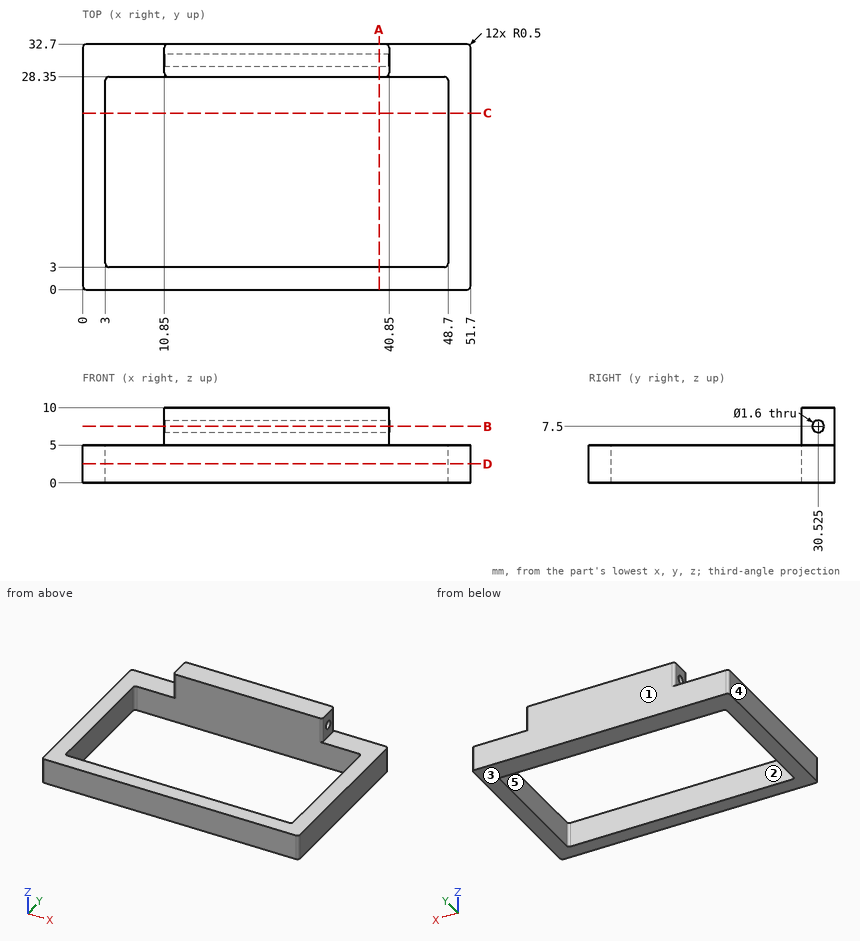
Geometry check sheet. Reference: drawing and pictorial views, mm from the part's lowest x, y, z. A direction names the side the tool comes from. Give positions to 0.01 mm unless a question says otherwise; leave off trailing zeros. Write each loop counter-clockwise with the first axis right and the second up, starting at its lowest first coordinate (ties: lowest second). Pieces come first, ordered by that corner, then holes. Notation, with made-up numbers: (-5, -38) - (28, -38) arc R17 cw to (28, -33) - close; hole circle Ø2 at (76, -36.75). An arc over 180 degrees is marked (long way). Put each result on its own line as item: value.
Q1. Mould release check, pull along Y, two halves, no side actions. Record for the marked faces 1, 2 and 3: released by +Y, released by -Y, zero draft, split by the parting line, or undercut.
Result:
face 1: released by +Y
face 2: undercut
face 3: zero draft
Q2. Section check B-B on z = 7.5. Record the cut outline in (x, y) (3 decimals).
Result:
outline: (10.85, 28.85) arc R0.5 ccw to (11.35, 28.35) - (40.35, 28.35) arc R0.5 ccw to (40.85, 28.85) - (40.85, 29.725) - (10.85, 29.725) - close; (10.85, 31.325) - (40.85, 31.325) - (40.85, 32.2) arc R0.5 ccw to (40.35, 32.7) - (11.35, 32.7) arc R0.5 ccw to (10.85, 32.2) - close
Q3. Section check A-A on x = 39.5. Record the cut outline in (y, z) (3 decimals).
Result:
outline: (0, 0) - (3, 0) - (3, 5) - (0, 5) - close; (28.35, 0) - (32.7, 0) - (32.7, 10) - (28.35, 10) - close; hole circle Ø1.6 at (30.525, 7.5)
Q4. Scan lines: probe 1 along Y at (x, z) = (37, 0.5); probe 2 along X at (y, z) = (8, 3.5); probe 3 along Y at (x, z) = (27.5, 9.5). Record each from-to range of solid material in increasing order. Write a range as from..to.
Result:
probe 1: 0..3, 28.35..32.7
probe 2: 0..3, 48.7..51.7
probe 3: 28.35..32.7
Q5. Section check C-C on y = 23.5. Record the cut outline in (x, z), and give its area (3 significant figures).
Result:
outline: (0, 0) - (3, 0) - (3, 5) - (0, 5) - close; (48.7, 0) - (51.7, 0) - (51.7, 5) - (48.7, 5) - close
area: 30.0 mm2
Q6. Section check D-D on z = 2.5. Record the cut outline in (x, y), and give its area (3 significant figures).
Result:
outline: (0, 0.5) arc R0.5 ccw to (0.5, 0) - (51.2, 0) arc R0.5 ccw to (51.7, 0.5) - (51.7, 32.2) arc R0.5 ccw to (51.2, 32.7) - (0.5, 32.7) arc R0.5 ccw to (0, 32.2) - close; hole (3, 3.5) arc R0.5 ccw to (3.5, 3) - (48.2, 3) arc R0.5 ccw to (48.7, 3.5) - (48.7, 27.85) arc R0.5 ccw to (48.2, 28.35) - (3.5, 28.35) arc R0.5 ccw to (3, 27.85) - close
area: 532 mm2
Q7. Depth check by flat-ended pin: P1, Ø1.5, axis at x = 19.5, z = 8.5, coming from the -Y side; P2, Ø1, axis at y = 30, z = 8.5, coming from the -X side; P3, Ø4, axis at x = 23.5, y = 5.5, coming from the +Z side; P4, Ø1, axis at y = 30.5, z = 6.5, coming from the +X side. Enter the tip coordinate at first touch or a pass-through.
Result:
P1: y = 28.35
P2: x = 10.85
P3: through
P4: x = 40.85
Q8. Set-up check for the marked faces 4 and 5: record each of +Z, -Z, +X, -X, +Y, -Y from which the full face is reachable in a straight line by a thin tool's end or side.
Result:
face 4: +Z, -Z, -X, +Y, -Y
face 5: +Z, -Z
